The model under review builds one solid part; all positions refer to its coordinate system, in mm. Face numbers are marked on the shaded views. A direction names the side the tool comes from. Give positions to 0.01 mm unless a question says otherwise; leave off trailing zeros. Order: outer loops, then holes, each group sorted by start corner. A loop starts at its lowest first (then second) coordinate and runs counter-clockwise, first axis right, second up.
```python
from build123d import *

# Parameters (mm, degrees)
BOSS_EXTRUDE1_DEPTH = 16
SKETCH2_R           = 4.25
CUT_EXTRUDE1_DEPTH  = 20
FILLET1_R           = 10
SKETCH3_R           = 40
CUT_EXTRUDE2_DEPTH  = 65.249513779
SKETCH5_R           = 40.5
SKETCH5_R_2         = 8
BOSS_EXTRUDE2_DEPTH = 5
BOSS_EXTRUDE3_START = 28
BOSS_EXTRUDE3_DEPTH = 28
SKETCH7_R           = 1.5
CUT_EXTRUDE3_DEPTH  = 71.434366784
CIRPATTERN1_COUNT   = 3
SKETCH8_R           = 1.65
CUT_EXTRUDE4_DEPTH  = 69.234888566
SKETCH9_R           = 3.5
CUT_EXTRUDE5_DEPTH  = 3
FILLET2_R           = 0.5
CUT_EXTRUDE6_DEPTH  = 69.234888566
CIRPATTERN2_COUNT   = 3
FILLET4_R           = 1


with BuildPart() as part:
    # Sketch1 → Boss-Extrude1 (new body)
    with BuildSketch(Plane(origin=(0, 0, 0), x_dir=(1, 0, 0), z_dir=(0, 1, 0))):
        with BuildLine():
            Line((-44, 0), (-44, -44))
            Line((-44, -44), (44, -44))
            Line((44, -44), (44, 0))
            ThreePointArc((44, 0), (0, 44), (-44, 0))
        make_face()
    extrude(amount=BOSS_EXTRUDE1_DEPTH)

    # Sketch2 → Cut-Extrude1 (cut)
    with BuildSketch(Plane.XY.offset(44)):
        with Locations((-38, 8)):
            Circle(SKETCH2_R)
        with Locations(Location((38, 8, 0), (0, 0, 180))):
            Circle(SKETCH2_R)
    extrude(amount=-CUT_EXTRUDE1_DEPTH, mode=Mode.SUBTRACT)

    # Fillet1
    # the kernel refuses this fillet: 10 mm, written as the material it takes off along each edge
    with BuildSketch(Plane(origin=(44, -25, 44), x_dir=(-1, 0, 0), z_dir=(0, 1, 0)), Plane(origin=(-44, -25, 44), x_dir=(0, 0, -1), z_dir=(0, 1, 0))) as fillet1_piece_1:
        with BuildLine():
            CenterArc((FILLET1_R, -FILLET1_R), FILLET1_R, 90, 90)
            Line((0, -FILLET1_R), (0, 0))
            Line((0, 0), (FILLET1_R, 0))
        make_face()
    extrude(amount=66, mode=Mode.SUBTRACT)

    # Sketch3 → Cut-Extrude2 (cut, through all)
    with BuildSketch(Plane(origin=(0, 16, 0), x_dir=(1, 0, 0), z_dir=(0, 1, 0))):
        with Locations(Location((0, 0, 0), (0, 0, 270))):
            Circle(SKETCH3_R)
    extrude(amount=-CUT_EXTRUDE2_DEPTH, mode=Mode.SUBTRACT)

    # Sketch5 → Boss-Extrude2 (add)
    with BuildSketch(Plane(origin=(0, 0, 0), x_dir=(1, 0, 0), z_dir=(0, 1, 0))):
        Circle(SKETCH5_R)
        with Locations(Location((0, 0, 0), (0, 0, 270))):
            Circle(SKETCH5_R_2, mode=Mode.SUBTRACT)
    extrude(amount=BOSS_EXTRUDE2_DEPTH)

    # Sketch6 → Boss-Extrude3 (add)
    with BuildSketch(Plane(origin=(0, 5, 0), x_dir=(1, 0, 0), z_dir=(0, 1, 0)).offset(BOSS_EXTRUDE3_START)):
        with BuildLine():
            Line((-13.680805733, 37.587704831), (-10.944644586, 30.070163865))
            ThreePointArc((-10.944644586, 30.070163865), (0, 32), (10.944644586, 30.070163865))
            Line((10.944644586, 30.070163865), (13.680805733, 37.587704831))
            ThreePointArc((13.680805733, 37.587704831), (0, 40), (-13.680805733, 37.587704831))
        make_face()
    boss_extrude3 = extrude(amount=-BOSS_EXTRUDE3_DEPTH)

    # Sketch7 → Cut-Extrude3 (cut, through all)
    with BuildSketch(Plane(origin=(0, 33, 0), x_dir=(1, 0, 0), z_dir=(0, 1, 0))):
        with Locations(Location((0, 36, 0), (0, 0, 270))):
            Circle(SKETCH7_R)
    cut_extrude3 = extrude(amount=-CUT_EXTRUDE3_DEPTH, mode=Mode.SUBTRACT)

    # CirPattern1: Boss-Extrude3, Cut-Extrude3 ×3 about axis
    cirpattern1_axis = Axis((0, 0, 0), (0, 1, 0))
    add([boss_extrude3.rotate(cirpattern1_axis, i * 360 / CIRPATTERN1_COUNT) for i in range(1, CIRPATTERN1_COUNT)])
    add([cut_extrude3.rotate(cirpattern1_axis, i * 360 / CIRPATTERN1_COUNT) for i in range(1, CIRPATTERN1_COUNT)], mode=Mode.SUBTRACT)

    # Sketch8 → Cut-Extrude4 (cut, through all)
    with BuildSketch(Plane(origin=(0, 5, 0), x_dir=(1, 0, 0), z_dir=(0, 1, 0))):
        with Locations(Location((-8.838834765, 8.838834765, 0), (0, 0, 270))):
            Circle(SKETCH8_R)
        with Locations(Location((8.838834765, 8.838834765, 0), (0, 0, 270))):
            Circle(SKETCH8_R)
        with Locations(Location((8.838834765, -8.838834765, 0), (0, 0, 270))):
            Circle(SKETCH8_R)
        with Locations(Location((-8.838834765, -8.838834765, 0), (0, 0, 270))):
            Circle(SKETCH8_R)
    extrude(amount=-CUT_EXTRUDE4_DEPTH, mode=Mode.SUBTRACT)

    # Sketch9 → Cut-Extrude5 (cut)
    with BuildSketch(Plane.XZ):
        with Locations(Location((8.838834765, 8.838834765, 0), (0, 0, 270))):
            Circle(SKETCH9_R)
        with Locations(Location((-8.838834765, 8.838834765, 0), (0, 0, 270))):
            Circle(SKETCH9_R)
        with Locations(Location((8.838834765, -8.838834765, 0), (0, 0, 270))):
            Circle(SKETCH9_R)
        with Locations(Location((-8.838834765, -8.838834765, 0), (0, 0, 270))):
            Circle(SKETCH9_R)
    extrude(amount=-CUT_EXTRUDE5_DEPTH, mode=Mode.SUBTRACT)

    # Fillet2
    fillet2_edges = [part.edges().sort_by_distance(p)[0] for p in [
        (-8.838834765, 0, 12.338834765),
        (8.838834765, 0, -5.338834765),
        (-8.838834765, 0, -5.338834765),
        (8.838834765, 0, 12.338834765),
    ]]
    fillet(fillet2_edges, radius=FILLET2_R)

    # Sketch10 → Cut-Extrude6 (cut, through all)
    with BuildSketch(Plane(origin=(0, 5, 0), x_dir=(1, 0, 0), z_dir=(0, 1, 0))):
        with BuildLine():
            ThreePointArc((13.680805733, 37.587704831), (14.309677586, 8.261696207), (39.39231012, -6.945927107))
            ThreePointArc((39.39231012, -6.945927107), (34.641016151, 20), (13.680805733, 37.587704831))
        make_face()
    cut_extrude6 = extrude(amount=-CUT_EXTRUDE6_DEPTH, mode=Mode.SUBTRACT)

    # CirPattern2: Cut-Extrude6 ×3 about axis
    cirpattern2_axis = Axis((0, 0, 0), (0, 1, 0))
    for i in range(1, CIRPATTERN2_COUNT):
        add(cut_extrude6.rotate(cirpattern2_axis, i * 360 / CIRPATTERN2_COUNT), mode=Mode.SUBTRACT)

    # Fillet4
    # the kernel refuses this fillet: 1 mm, written as the material it takes off along each edge
    with BuildSketch(Plane(origin=(13.680805733, 35.56431335, -37.587704831), x_dir=(-0.3420201433256679, 0, 0.9396926207859085), z_dir=(0, -1, 0)), Plane(origin=(-39.39231012, 35.56431335, 6.945927107), x_dir=(0.9848077530122079, 0, -0.17364817766693066), z_dir=(0, -1, 0))) as fillet4_piece_1:
        with BuildLine():
            CenterArc((1.012822621, 1), FILLET4_R, 178.530716419, 91.469283581)
            ThreePointArc((0.013151406, 1.025641026), (0.003287987, 0.51286267), (0, 0))
            Line((0, 0), (1.012822621, 0))
        make_face()
    extrude(amount=19.56431335, mode=Mode.SUBTRACT)
    with BuildSketch(Plane(origin=(-13.680805733, 35.56431335, -37.587704831), x_dir=(0.3420201433256646, 0, 0.93969262078591), z_dir=(0, -1, 0)), Plane(origin=(39.39231012, 35.56431335, 6.945927107), x_dir=(-0.984807753012207, 0, -0.17364817766693638), z_dir=(0, -1, 0))) as fillet4_piece_2:
        with BuildLine():
            CenterArc((1.012822621, -1), FILLET4_R, 90, 91.469283581)
            ThreePointArc((0.013151406, -1.025641026), (0.003287987, -0.51286267), (0, 0))
            Line((0, 0), (1.012822621, 0))
        make_face()
    extrude(amount=19.56431335, mode=Mode.SUBTRACT)
    with BuildSketch(Plane(origin=(-10.944644586, 35.462112512, -30.070163865), x_dir=(-0.34202014332566283, 0, -0.9396926207859105), z_dir=(0, -1, 0)), Plane(origin=(-20.56920351, 35.462112512, 24.51342218), x_dir=(-0.6427876096865429, 0, 0.766044443118975), z_dir=(0, -1, 0)), Plane(origin=(31.513848096, 35.462112512, 5.556741685), x_dir=(0.984807753012207, 0, 0.1736481776669362), z_dir=(0, -1, 0))) as fillet4_piece_3:
        with BuildLine():
            CenterArc((0.984845005, 1), FILLET4_R, 181.736501576, 88.263498424)
            ThreePointArc((-0.014695753, 0.96969697), (-0.003674149, 0.48490416), (0, 0))
            Line((0, 0), (0.984845005, 0))
        make_face()
    extrude(amount=30.462112512, mode=Mode.SUBTRACT)
    with BuildSketch(Plane(origin=(10.944644586, 35.462112512, -30.070163865), x_dir=(0.34202014332566955, 0, -0.9396926207859082), z_dir=(0, -1, 0)), Plane(origin=(-31.513848096, 35.462112512, 5.556741685), x_dir=(-0.9848077530122084, 0, 0.17364817766692914), z_dir=(0, -1, 0)), Plane(origin=(20.56920351, 35.462112512, 24.51342218), x_dir=(0.6427876096865386, 0, 0.7660444431189787), z_dir=(0, -1, 0))) as fillet4_piece_4:
        with BuildLine():
            CenterArc((0.984845005, -1), FILLET4_R, 90, 88.263498424)
            ThreePointArc((-0.014695753, -0.96969697), (-0.003674149, -0.48490416), (0, 0))
            Line((0, 0), (0.984845005, 0))
        make_face()
    extrude(amount=30.462112512, mode=Mode.SUBTRACT)
    with BuildSketch(Plane(origin=(-25.711504387, 35.56431335, 30.641777725), x_dir=(-0.7577399302790805, 0, -0.6525566627202992), z_dir=(0, -1, 0))) as fillet4_piece_5:
        with BuildLine():
            CenterArc((1.012903773, 0.9999178), FILLET4_R, 179.265358209, 91.469283581)
            Line((0.012985973, 1.012739367), (0, 0))
            ThreePointArc((0, 0), (0.51286267, -0.003287987), (1.02572534, 0))
        make_face()
    extrude(amount=19.56431335, mode=Mode.SUBTRACT)
    with BuildSketch(Plane(origin=(25.711504387, 35.56431335, 30.641777725), x_dir=(0.7577399302790873, 0, -0.6525566627202912), z_dir=(0, -1, 0))) as fillet4_piece_6:
        with BuildLine():
            CenterArc((1.012903773, -0.9999178), FILLET4_R, 89.265358209, 91.469283581)
            Line((0.012985973, -1.012739367), (0, 0))
            ThreePointArc((0, 0), (0.51286267, 0.003287987), (1.02572534, 0))
        make_face()
    extrude(amount=19.56431335, mode=Mode.SUBTRACT)


solid = part.part
```
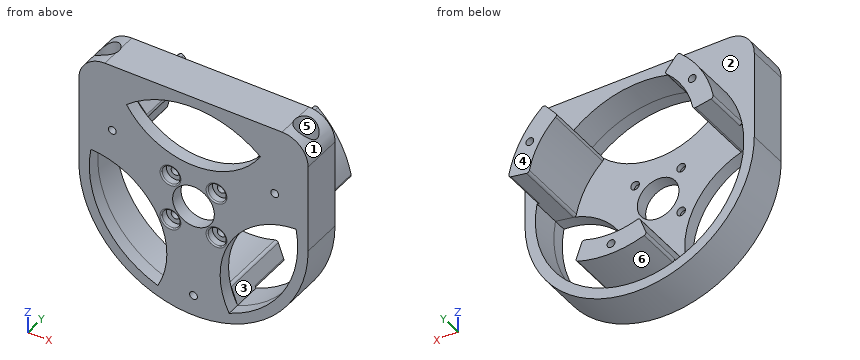
1. Draft analysis for pull direction X (two halves, no side actions). For the marked faces 4, 5 and 6, state which applies: pulls with the +X half, pulls with the -X half, needs draft (parallel to the pull), parting line crosses it, or undercut.
2. For the marked faces 1, 2 and 3, list the 3-axis set-ups (+Z, -Z, +X, -X, +Y, -Y) from which the entire face can be reached by the end or side of a thin tool; tool diameter is ignored.
3. To check wall thickness, follow line 1 (X direction, y = 7.5, z = 18); line 2 (X direction, y = 8, z = 35.5); line 3 (Y direction, x = -30.5, z = 36.5). State the ranges of each line that lie inside material, in increasing order.
4. Take a section at A-A (x = 0). Write out the cut boundary in (y, z), and give its area (3 significant figures).
5. Take a section at C-C (x = -19). Write out the cut boundary in (y, z), and give its area (3 significant figures).
6. Take a section at B-B (y = 30). Write out the cut boundary in (x, z).
7. Take a section at D-D (y = 13.5). Write out the cut boundary in (x, z), and give its area (3 significant figures).
8. Insertion check: pin 1 (3.5 mm diameter, centred on x = 9, z = -8.5, fed in from -Y); pin 2 (8 mm diameter, centred on x = -8.84, z = -8.84, fed in from +Y); pin 3 (6 mm diameter, centred on y = 26, z = 19.5, fed in from +X). Each pin has a flat end and moves straight along its axis. Give the tip position at first contact, or say it passes through.
Answer:
1. face 4: needs draft
1. face 5: undercut
1. face 6: parting line crosses it
2. face 1: +Z, +X, +Y, -Y
2. face 2: +Y
2. face 3: +Y, -Y
3. line 1: x = -44 to -32.68, -29.68 to -26.46, 26.46 to 29.68, 32.68 to 44
3. line 2: x = -43.89 to -42.25, -33.75 to -18.43, 18.43 to 33.75, 42.25 to 43.89
3. line 3: y = 0 to 16
4. outline: (0, -44) - (16, -44) - (16, -40) - (33, -40) - (33, -37.5) - (0, -37.5) - close; (0, -34.5) - (33, -34.5) - (33, -32) - (5, -32) - (5, -8) - (0, -8) - close; (0, 8) - (5, 8) - (5, 16.52) - (0, 16.52) - close; (0, 40) - (16, 40) - (16, 44) - (0, 44) - close
4. area: 456 mm2
5. outline: (0, -39.69) - (16, -39.69) - (16, -35.2) - (0, -35.2) - close; (0, -2.1) - (5, -2.1) - (5, 23.17) - (0, 23.17) - close; (0, 35.2) - (16, 35.2) - (16, 44) - (0, 44) - close
5. area: 339 mm2
6. outline: (-39.2, 7.95) arc R1 ccw to (-38.39, 6.77) - (-32.48, 5.73) arc R1 ccw to (-31.33, 6.51) arc R32 cw to (-21.3, 23.88) arc R1 ccw to (-21.2, 25.27) - (-25.06, 29.87) arc R1 ccw to (-26.49, 29.97) arc R40 ccw to start; (-13.33, -36.64) arc R1 ccw to (-12.71, -37.93) arc R40 ccw to (12.71, -37.93) arc R1 ccw to (13.33, -36.64) - (11.28, -31) arc R1 ccw to (10.03, -30.39) arc R32 cw to (-10.03, -30.39) arc R1 ccw to (-11.28, -31) - close; (21.2, 25.27) arc R1 ccw to (21.3, 23.88) arc R32 cw to (31.33, 6.51) arc R1 ccw to (32.48, 5.73) - (38.39, 6.77) arc R1 ccw to (39.2, 7.95) arc R40 ccw to (26.49, 29.97) arc R1 ccw to (25.06, 29.87) - close; hole circle Ø3 at (-31.18, 18); hole circle Ø3 at (0, -36); hole circle Ø3 at (31.18, 18)
7. outline: (-44, 0) arc R44 ccw to (44, 0) - (44, 34) arc R10 ccw to (34, 44) - (-34, 44) arc R10 ccw to (-44, 34) - close; hole (-39.39, 6.95) arc R40 ccw to (-13.68, -37.59) - (-11.28, -31) arc R1 cw to (-10.03, -30.39) arc R32 ccw to (10.03, -30.39) arc R1 cw to (11.28, -31) - (13.68, -37.59) arc R40 ccw to (39.39, 6.95) - (32.48, 5.73) arc R1 cw to (31.33, 6.51) arc R32 ccw to (21.3, 23.88) arc R1 cw to (21.2, 25.27) - (25.71, 30.64) arc R40 ccw to (-25.71, 30.64) - (-21.2, 25.27) arc R1 cw to (-21.3, 23.88) arc R32 ccw to (-31.33, 6.51) arc R1 cw to (-32.48, 5.73) - close; hole circle Ø3 at (-31.18, 18); hole circle Ø3 at (0, -36); hole circle Ø3 at (31.18, 18)
7. area: 2,420 mm2
8. pin 1: stops at y = 3
8. pin 2: stops at y = 5
8. pin 3: stops at x = 36.44
